Here's how the part is built. I have some questions about the finished solid (model axes, mm). A direction names the side the tool comes from. Round coordinates to 2 decimals unless told otherwise and drop trailing zeros. Write each loop counter-clockwise with the first axis right and the second up, starting at its lowest first coordinate (ties: lowest second). Pieces come first, ordered by that corner, then holes. Notation, with made-up numbers: (-12.75, 46.5) - (15.25, 46.5) arc R34 ccw to (15.25, 79.5) - close; hole circle Ø3 at (70, 68.5). An arc over 180 degrees is marked (long way). Use one line per item in the form item = value. Start each with the question number.
1. I want a section at B-B, the plane y = -5.75. List the corners of the cut face in (x, z) for me, plus the area to 3 significant figures.
2. Which directions (+Z, -Z, +X, -X, +Y, -Y) give clear straight access to the entire face, cutting with the end or side of a thin tool? Please do faces 3 (the flat face through (0, 1.75, -1)), 4 (the flat face through (-21, -2.15, 30)), 5 (the flat face through (-28.05, -1, 0)).
3. We'd pull the mould along X, two halves only. Please class faces 1 (the flat face through (0, 1.75, -33)), 2 (the flat face through (-20.902, -2.094, 27.989)): +X half, -X half, draft (parallel to the pull), parting line (faces both ways), or undercut.
4. Will these pins go through, and if not, where does the flat tip stop? pin 1 (1.4 mm diameter, centred on x = 6, z = -5, fed in from +Y); pin 2 (1.5 mm diameter, centred on x = 12.5, z = -27, fed in from -Y); pin 3 (5 mm diameter, centred on x = -8, z = -15, fed in from -Y).
5. I want a section at A-A, the plane z = 24. List the corners of the cut face in (x, y) for me, plus the area to 3 significant figures.
6. If I drill on line 1 along Z through (x, y) = (17, -1.25); line 2 along Z through (x, y) = (-2, 1.25); line 3 along Z through (x, y) = (2, -1.25), over which ranges is the centre line in solid material (lowest first)?
```python
from build123d import *

# Parameters (mm, degrees)
SKETCH1_W           = 60.6
SKETCH1_H           = 58.5
BOSS_EXTRUDE1_DEPTH = 2
SKETCH2_W           = 56.1
SKETCH2_H           = 23.5
SKETCH2_H_2         = 14
CUT_EXTRUDE1_DEPTH  = 1.5
CUT_EXTRUDE2_REACH  = 67.912
SKETCH3_W           = 56.1
SKETCH3_H           = 1.25
BOSS_EXTRUDE2_START = 17.5
BOSS_EXTRUDE2_DEPTH = 6.9
BOSS_EXTRUDE3_DEPTH = 6
DRAFT1_START        = -35
DRAFT1_DEPTH        = 5.75
FILLET1_R           = 0.45
FILLET2_R           = 0.602786
FILLET3_R           = 1.418858
FILLET4_R           = 1
SKETCH6_W           = 57.6
SKETCH6_H           = 1.75
CUT_EXTRUDE3_DEPTH  = 0.25
CHAMFER1_START      = 25.032204955
CHAMFER1_OUTLINE_W  = 60.6
CHAMFER1_OUTLINE_H  = 3
CHAMFER1_DEPTH      = 1.967795045
FILLET5_START       = -31
FILLET5_DEPTH       = 62
FILLET6_R           = 0.25
CUT_SWEEP1_START    = -31
CUT_SWEEP1_DEPTH    = 0.95
CUT_SWEEP1_START_2  = 30.05
CUT_SWEEP1_2_DEPTH  = 0.95


with BuildPart() as part:
    # Sketch1 → Boss-Extrude1 (new, symmetric)
    with BuildSketch(Plane(origin=(0, 0, 0), x_dir=(1, 0, 0), z_dir=(0, 1, 0))):
        Rectangle(SKETCH1_W, SKETCH1_H)
    extrude(amount=BOSS_EXTRUDE1_DEPTH, both=True)

    # Sketch2 → Cut-Extrude1 (cut)
    with BuildSketch(Plane.XZ.offset(2)):
        Rectangle(SKETCH2_W, SKETCH2_H)
        with Locations((0, 20.25)):
            Rectangle(SKETCH2_W, SKETCH2_H_2)
        with Locations((0, -20.25)):
            Rectangle(SKETCH2_W, SKETCH2_H_2)
    extrude(amount=-CUT_EXTRUDE1_DEPTH, mode=Mode.SUBTRACT)

    # Sketch3 → Cut-Extrude2 (cut, up to next)
    with BuildSketch(Plane(origin=(0, 0, -29.25), x_dir=(-1, 0, 0), z_dir=(0, 0, -1)), mode=Mode.PRIVATE) as cut_extrude2_sk1:
        with Locations((0, -1.375)):
            Rectangle(SKETCH3_W, SKETCH3_H)
    cut_extrude2_tool1 = extrude(cut_extrude2_sk1.sketch, amount=-CUT_EXTRUDE2_REACH, mode=Mode.PRIVATE) & part.part
    cut_extrude2 = cut_extrude2_tool1.solids().sort_by_distance((0, -1.375, -29.25))[0]
    add(cut_extrude2, mode=Mode.SUBTRACT)

    # Mirror1: Cut-Extrude2 across plane
    add(cut_extrude2.mirror(Plane.XY), mode=Mode.SUBTRACT)

    # Boss-Extrude2: read off the stored shape, not the designer's step
    # Boss-Extrude2 outline → Boss-Extrude2 (add)
    with BuildSketch(Plane.YZ.offset(BOSS_EXTRUDE2_START)):
        Polygon((-0.75, 29.25), (-2.15, 29.25), (-2.15, 30.669097299), (-3.4, 30.614521121), (-3.4, 28.464521121), (-0.75, 27.5), align=None)
    boss_extrude2 = extrude(amount=BOSS_EXTRUDE2_DEPTH)

    # Sketch5 → Boss-Extrude3 (add, symmetric)
    with BuildSketch(Plane(origin=(0, 0, 0), x_dir=(0, 0, -1), z_dir=(1, 0, 0))):
        Polygon((29.25, 1.5), (30.25, 1.5), (30.25, -9.75), (31.357502325, -9.75), (32.25, -4.75), (32.25, 1.75), (34.25, 1.75), (34.25, 0.85), (33.65, 0.85), (33.65, -4.5), (32.024952176, -11.25), (29.524952176, -11.25), (29.25, -0.75), align=None)
    extrude(amount=BOSS_EXTRUDE3_DEPTH, both=True)

    # Draft1: read off the stored shape, not the designer's step
    # Draft1 outline → Draft1 (cut)
    with BuildSketch(Plane.XY.offset(DRAFT1_START)):
        Polygon((5.305596924, -11.25), (6, -11.25), (6, 1.75), (5.986898055, 1.75), align=None)
        Polygon((-6, -11.25), (-5.305596924, -11.25), (-5.986898055, 1.75), (-6, 1.75), align=None)
    extrude(amount=DRAFT1_DEPTH, mode=Mode.SUBTRACT)

    # Fillet1
    fillet1_edges = [part.edges().sort_by_distance(p)[0] for p in [
        (0, 0.85, -34.25),
        (0, 1.75, -34.25),
    ]]
    fillet(fillet1_edges, radius=FILLET1_R - 0.0001)  # a hair under: the kernel refuses the full size

    # Fillet2
    fillet2_edges = [part.edges().sort_by_distance(p)[0] for p in [
        (0, -9.75, -31.357502325),
        (0, -9.75, -30.25),
    ]]
    fillet(fillet2_edges, radius=FILLET2_R - 0.0001)  # a hair under: the kernel refuses the full size

    # Fillet3
    fillet3_edges = [part.edges().sort_by_distance(p)[0] for p in [
        (0, -11.25, -29.524952176),
        (0, -11.25, -32.024952176),
    ]]
    fillet(fillet3_edges, radius=FILLET3_R - 0.0001)  # a hair under: the kernel refuses the full size

    # Fillet4
    fillet4_edges = [part.edges().sort_by_distance(p)[0] for p in [
        (0, -0.75, -29.25),
    ]]
    fillet(fillet4_edges, radius=FILLET4_R)

    # Sketch6 → Cut-Extrude3 (cut)
    with BuildSketch(Plane(origin=(0, 2, 0), x_dir=(1, 0, 0), z_dir=(0, 1, 0))):
        with Locations((0, 27.625)):
            Rectangle(SKETCH6_W, SKETCH6_H)
        with Locations((0, 23.125)):
            Rectangle(SKETCH6_W, SKETCH6_H)
        with Locations((0, 18.625)):
            Rectangle(SKETCH6_W, SKETCH6_H)
        with Locations((0, 14.125)):
            Rectangle(SKETCH6_W, SKETCH6_H)
        with Locations((0, 9.625)):
            Rectangle(SKETCH6_W, SKETCH6_H)
        with Locations((0, 5.125)):
            Rectangle(SKETCH6_W, SKETCH6_H)
        with Locations((0, 0.625)):
            Rectangle(SKETCH6_W, SKETCH6_H)
        with Locations((0, -3.875)):
            Rectangle(SKETCH6_W, SKETCH6_H)
        with Locations((0, -8.375)):
            Rectangle(SKETCH6_W, SKETCH6_H)
        with Locations((0, -12.875)):
            Rectangle(SKETCH6_W, SKETCH6_H)
    extrude(amount=-CUT_EXTRUDE3_DEPTH, mode=Mode.SUBTRACT)

    # Chamfer1: read off the stored shape, not the designer's step
    # Chamfer1 outline → Chamfer1 (cut)
    with BuildSketch(Plane(origin=(0, 0, 0), x_dir=(1, 0, 0), z_dir=(0, 0.500000000000001, 0.866025403784438)).offset(CHAMFER1_START)):
        with Locations((0, -13.642949192)):
            Rectangle(CHAMFER1_OUTLINE_W, CHAMFER1_OUTLINE_H)
    extrude(amount=CHAMFER1_DEPTH, mode=Mode.SUBTRACT)

    # Fillet5: read off the stored shape, not the designer's step
    # Fillet5 outline → Fillet5 (cut)
    with BuildSketch(Plane.YZ.offset(FILLET5_START)):
        with BuildLine():
            ThreePointArc((1.25, 28.183012702), (1.799038106, 27.633974596), (2, 26.883974596))
            Line((2, 26.883974596), (2, 27.75))
            Line((2, 27.75), (1.25, 28.183012702))
        make_face()
    extrude(amount=FILLET5_DEPTH, mode=Mode.SUBTRACT)

    # Fillet6
    fillet6_edges = [part.edges().sort_by_distance(p)[0] for p in [
        (0, -0.598076211, 29.25),
    ]]
    fillet(fillet6_edges, radius=FILLET6_R)

    # Cut-Sweep1: read off the stored shape, not the designer's step
    # Cut-Sweep1 outline → Cut-Sweep1 (cut)
    with BuildSketch(Plane.YZ.offset(CUT_SWEEP1_START)):
        with BuildLine():
            ThreePointArc((1.125, 27.966506351), (1.582531755, 27.508974596), (1.75, 26.883974596))
            Line((1.75, 26.883974596), (1.75, -29.25))
            Line((1.75, -29.25), (2, -29.25))
            Line((2, -29.25), (2, 26.883974596))
            ThreePointArc((2, 26.883974596), (1.799038106, 27.633974596), (1.25, 28.183012702))
            Line((1.25, 28.183012702), (-0.540063509, 29.216506351))
            ThreePointArc((-0.540063509, 29.216506351), (-0.600358748, 29.241481457), (-0.665063509, 29.25))
            Line((-0.665063509, 29.25), (-2, 29.25))
            Line((-2, 29.25), (-2, 29))
            Line((-2, 29), (-0.665063509, 29))
            Line((-0.665063509, 29), (1.125, 27.966506351))
        make_face()
    extrude(amount=CUT_SWEEP1_DEPTH, mode=Mode.SUBTRACT)

    # Cut-Sweep1 2 outline → Cut-Sweep1 2 (cut)
    with BuildSketch(Plane.YZ.offset(CUT_SWEEP1_START_2)):
        with BuildLine():
            ThreePointArc((1.125, 27.966506351), (1.582531755, 27.508974596), (1.75, 26.883974596))
            Line((1.75, 26.883974596), (1.75, -29.25))
            Line((1.75, -29.25), (2, -29.25))
            Line((2, -29.25), (2, 26.883974596))
            ThreePointArc((2, 26.883974596), (1.799038106, 27.633974596), (1.25, 28.183012702))
            Line((1.25, 28.183012702), (-0.540063509, 29.216506351))
            ThreePointArc((-0.540063509, 29.216506351), (-0.600358748, 29.241481457), (-0.665063509, 29.25))
            Line((-0.665063509, 29.25), (-2, 29.25))
            Line((-2, 29.25), (-2, 29))
            Line((-2, 29), (-0.665063509, 29))
            Line((-0.665063509, 29), (1.125, 27.966506351))
        make_face()
    extrude(amount=CUT_SWEEP1_2_DEPTH, mode=Mode.SUBTRACT)

    # Mirror2: Boss-Extrude2 across plane
    add(boss_extrude2.mirror(Plane(origin=(0, 0, 0), x_dir=(0, 0, 1), z_dir=(1, 0, 0))))


solid = part.part
```
Model answer:
q1.outline = (-5.59, -33.35) - (5.59, -33.35) - (5.59, -32.07) - (-5.59, -32.07) - close; (-5.59, -30.25) - (5.59, -30.25) - (5.59, -29.38) - (-5.59, -29.38) - close
q1.area = 24.0 mm2
q2.face_3 = +Y
q2.face_4 = +Z, +X, -X, +Y
q2.face_5 = -Y
q3.face_1 = draft
q3.face_2 = undercut
q4.pin_1 = 1.75
q4.pin_2 = -0.75
q4.pin_3 = -2
q5.outline = (-30.3, -2) - (-28.05, -2) - (-28.05, -0.5) - (28.05, -0.5) - (28.05, -2) - (30.3, -2) - (30.3, 1.75) - (30.05, 1.75) - (30.05, 2) - (-30.05, 2) - (-30.05, 1.75) - (-30.3, 1.75) - close
q5.area = 158 mm2
q6.line_1 = -13.25 to -11.75, 11.75 to 13.25
q6.line_2 = -34.25 to -32.25, -30.25 to 28.18
q6.line_3 = -33.65 to -32.25, -30.25 to -29.14, -13.25 to -11.75, 11.75 to 13.25
